Source: CAD feature listing. Evaluate the final solid. Frame: model axes, mm. A direction names the side the tool comes from. Round coordinates to 2 decimals unless told otherwise and drop trailing zeros. Write each loop counter-clockwise with the first axis right and the second up, starting at its lowest first coordinate (ties: lowest second). Pieces come first, ordered by that corner, then holes. Notation, with made-up numbers: M 83,-24.5 L 98,-24.5 A12 cw 98,-13.5 Z; hole C 33.5,21 d1. An arc over 180 degrees is marked long. Answer in a Markdown table with one row per item.
from build123d import *

# Parameters (mm, degrees)
F0_W     = 542.360485
F0_H     = 168.78362
F1_DEPTH = 25.4
F2_R     = 25.4
F3_R     = 5.08
F4_R     = 40.946122
F4_R_2   = 31.465149
F5_DEPTH = 25.4


with BuildPart() as f1:
    # F0 (on Front) → F1 (new body)
    with BuildSketch(Plane.XZ):
        with Locations((176.964849, -1.053691)):
            Rectangle(F0_W, F0_H)
        with BuildLine():
            ThreePointArc((54.161403, -16.155303), (-56.51663, 0.567409), (54.474841, 15.064629))
            Line((54.474841, 15.064629), (118.513588, 15.064629))
            ThreePointArc((118.513588, 15.064629), (145.08589, 22.54609), (161.0149, 0))
            ThreePointArc((161.0149, 0), (145.760851, -22.295352), (119.453656, -16.155303))
            Line((119.453656, -16.155303), (54.161403, -16.155303))
        make_face(mode=Mode.SUBTRACT)
    extrude(amount=F1_DEPTH)

    # F2
    f2_edges = [f1.edges().sort_by_distance(p)[0] for p in [
        (448.145092, -12.7, 83.338119),
        (448.145092, -12.7, -85.445501),
        (-94.215393, -12.7, 83.338119),
        (-94.215393, -12.7, -85.445501),
    ]]
    fillet(f2_edges, radius=F2_R)

    # F3
    f3_edges = [f1.edges().sort_by_distance(p)[0] for p in [
        (54.474841, -12.7, 15.064629),
        (119.453656, -12.7, -16.155303),
        (54.161403, -12.7, -16.155303),
        (118.513588, -12.7, 15.064629),
    ]]
    fillet(f3_edges, radius=F3_R)

    # F4 (on face) → F5 (cut)
    with BuildSketch(Plane.XZ.offset(25.4)):
        with Locations((244.522035, 0)):
            Circle(F4_R)
        with Locations((368.218273, 0)):
            Circle(F4_R_2)
    extrude(amount=-F5_DEPTH, mode=Mode.SUBTRACT)


solid = f1.part
Q1. Access query for faces 5 (the flat face through (173, 0, 0)), 6 (the flat face through (87, -13, 15.065)). Directions: +Z, -Z, +X, -X, +Y, -Y. A direction counts if a zero-diameter tool reaches every point of the face in a straight line with its end or side. Return the directions, or none.
Solutions:
| item | result |
|---|---|
| face 5 | +Z, -Z, +X, -X, +Y |
| face 6 | +Y, -Y |
Q2. Pull-direction query (Z, two-part tool) for faces 1 (the flat face through (174, -13, 83.338)), 2 (the flat face through (88, -13, -16.155)), 3 (the cylindrical face through (343.25, -12.88, -19.15)), 4 (the flat face through (174, -13, -85.446)); classes: pulls with the +Z half, pulls with the -Z half, needs draft (parallel to the pull), parting line crosses it, or undercut.
Solutions:
| item | result |
|---|---|
| face 1 | pulls with the +Z half |
| face 2 | undercut |
| face 3 | undercut |
| face 4 | pulls with the -Z half |
Q3. Material intervals for probe 1 along Z at (x, y) = (64, -21.5); probe 2 along X at (y, z) = (-6, 2.5); probe 3 along X at (y, z) = (-22, -9), sorted ascending.
Solutions:
| item | result |
|---|---|
| probe 1 | z = -85.45 to -16.16, 15.06 to 83.34 |
| probe 2 | x = -94.22 to -56.46, 160.88 to 203.65, 285.39 to 336.85, 399.58 to 448.15 |
| probe 3 | x = -94.22 to -55.8, 159.26 to 204.58, 284.47 to 338.07, 398.37 to 448.15 |
Q4. Section C-C (x = 129). Return loops of the section in (y, z).
Solutions:
| item | result |
|---|---|
| outline | M -25.4,-85.45 L 0,-85.45 L 0,-22.51 L -25.4,-22.51 Z; M -25.4,22.51 L 0,22.51 L 0,83.34 L -25.4,83.34 Z |
Q5. Section B-B (y = -9). Return loops of the section in (x, z), and give its area (3 significant figures).
Solutions:
| item | result |
|---|---|
| outline | M -94.22,-60.05 A25.4 ccw -68.82,-85.45 L 422.75,-85.45 A25.4 ccw 448.15,-60.05 L 448.15,57.94 A25.4 ccw 422.75,83.34 L -68.82,83.34 A25.4 ccw -94.22,57.94 Z; hole M 53.05,-19.48 A5.08 cw 57.82,-16.16 L 117.34,-16.16 A5.08 cw 120.8,-17.52 A23.92 ccw 161.01,0 A23.92 ccw 119.89,16.62 A5.08 cw 116.23,15.06 L 58.21,15.06 A5.08 cw 53.41,18.48 A56.52 ccw long Z; hole C 244.52,0 d81.89; hole C 368.22,0 d62.93 |
| area | 68,900 mm2 |
Q6. Section A-A (x = 0). Return loops of the section in (y, z), and give its area (3 significant figures).
Solutions:
| item | result |
|---|---|
| outline | M -25.4,-85.45 L 0,-85.45 L 0,-56.52 L -25.4,-56.52 Z; M -25.4,56.52 L 0,56.52 L 0,83.34 L -25.4,83.34 Z |
| area | 1,420 mm2 |
